Input: part model. Units: mm. Frame: model coordinates. A direction names the side the tool comes from. Coordinates: 2 decimals unless noted, no trailing zeros. Loops run counter-clockwise (first coordinate to the right, second up) from the corner with the lowest first, then second, coordinate; pieces in that order, holes last.
Item 1: Section C-C on z = 1.5. Give the number of separate pieces and of enclosed holes in the cut face, and give its area (3 significant figures).
Item 2: Ray query, line 1 along Z through (x, y) = (10, 0.55) (3 decimals); line 2 along Z through (x, y) = (0, 2.75); line 3 along X through (y, z) = (4.5, 0.75). Return the intervals inside material, ascending.
Item 3: Section D-D on y = 6.5. Return loops of the section in (x, z).
Item 4: Reachability of faces 5 (the flat face through (5, 7, 0)), 6 (the flat face through (0, 5, 2)) from +Z, -Z, +X, -X, +Y, -Y: full face, straight path, thin tool, end or side. Return the list, or none.
Item 5: Pull-direction query (Z, two-part tool) for faces 1 (the flat face through (12.5, 4.54, 1.47)), 2 (the flat face through (5, 3, -5)), 3 (the cylindrical face through (15, 3, 0)), 4 (the flat face through (7.477, 4.535, 1.43)); classes: released by +Z, released by -Z, zero draft, split by the parting line, or undercut.
Item 6: Section A-A on y = 2.25. Return loops of the section in (x, z).
Item 7: Section B-B on x = 9.75. Return loops of the section in (y, z).
Item 8: Contact query for flat-ended pins moving along their axis: P1, Ø1.5, axis at x = 11, y = 4.5, coming from the -Z side; P2, Ø2.5, axis at x = 0, z = 0, coming from the +Y side. Output: stop coordinate, or through.
```python
from build123d import *

# Parameters (mm, degrees)
EXTRUDE_2_DEPTH              = 7
CUT_EXTRUDE_1_DEPTH          = 4
HOLE_WIZARD_M3_1_D           = 3.4
HOLE_WIZARD_M3_1_CSINK_D     = 6.72
HOLE_WIZARD_M3_1_CSINK_ANGLE = 90
HOLE_WIZARD_1_D              = 4.15
HOLE_WIZARD_1_DEPTH          = 10
CUT_EXTRUDE_2_DEPTH          = 5


with BuildPart() as part:
    # 草图1 → 凸台-拉伸2 (new body)
    with BuildSketch(Plane(origin=(0, 0, 0), x_dir=(1, 0, 0), z_dir=(0, 1, 0))):
        with BuildLine():
            Line((0, 5), (10, 5))
            ThreePointArc((10, 5), (15, 0), (10, -5))
            Line((10, -5), (0, -5))
            ThreePointArc((0, -5), (-5, 0), (0, 5))
        make_face()
    extrude(amount=EXTRUDE_2_DEPTH)

    # 草图2 → 切除-拉伸1 (cut)
    with BuildSketch(Plane(origin=(0, 7, 0), x_dir=(1, 0, 0), z_dir=(0, 1, 0))):
        with BuildLine():
            Line((1.5, 2), (-1.5, 2))
            ThreePointArc((-1.5, 2), (-2.5, 0), (-1.5, -2))
            Line((-1.5, -2), (1.5, -2))
            ThreePointArc((1.5, -2), (2.236067977, -1.118033989), (2.5, 0))
            ThreePointArc((2.5, 0), (2.236067977, 1.118033989), (1.5, 2))
        make_face()
    extrude(amount=-CUT_EXTRUDE_1_DEPTH, mode=Mode.SUBTRACT)

    # M3 六角凹锥坑螺钉的锥形沉头孔1 (through all)
    with Locations(Plane(origin=(0, 0, 0), x_dir=(-1, 0, 0), z_dir=(0, -1, 0))):
        with Locations((0, 0)):
            CounterSinkHole(HOLE_WIZARD_M3_1_D / 2, HOLE_WIZARD_M3_1_CSINK_D / 2, counter_sink_angle=HOLE_WIZARD_M3_1_CSINK_ANGLE)

    # 孔1
    with Locations(Plane(origin=(0, 7, 0), x_dir=(1, 0, 0), z_dir=(0, 1, 0))):
        with Locations((10, 0)):
            Hole(HOLE_WIZARD_1_D / 2, depth=HOLE_WIZARD_1_DEPTH)

    # 草图8 → 切除-拉伸2 (cut)
    with BuildSketch(Plane(origin=(0, 7, 0), x_dir=(1, 0, 0), z_dir=(0, 1, 0))):
        Polygon((13.348631561, 0), (11.674315781, 2.9), (8.325684219, 2.9), (6.651368439, 0), (8.325684219, -2.9), (11.674315781, -2.9), align=None)
    extrude(amount=-CUT_EXTRUDE_2_DEPTH, mode=Mode.SUBTRACT)


solid = part.part
```
Results found:
1. separate pieces: 3
1. enclosed holes: 0
1. area: 81.4 mm2
2. line 1: z = -5 to -2.075, 2.075 to 5
2. line 2: z = -5 to -1.7, 1.7 to 5
2. line 3: x = -4.94 to -2.38, 2.38 to 7.08, 12.92 to 14.94
3. outline: (0, -5) - (10, -5) arc R5 ccw to (10, 5) - (0, 5) arc R5 ccw to start; hole (-1.5, -2) - (1.5, -2) arc R2.5 ccw to (1.5, 2) - (-1.5, 2) arc R2.5 ccw to start; hole (6.65, 0) - (8.33, -2.9) - (11.67, -2.9) - (13.35, 0) - (11.67, 2.9) - (8.33, 2.9) - close
4. face 5: +Z, -Z, +X, -X, +Y
4. face 6: +Y
5. face 1: undercut
5. face 2: released by -Z
5. face 3: split by the parting line
5. face 4: undercut
6. outline: (0, -5) - (10, -5) arc R5 ccw to (10, 5) - (0, 5) arc R5 ccw to start; hole circle Ø3.4 at (0, 0); hole (6.65, 0) - (8.33, -2.9) - (11.67, -2.9) - (13.35, 0) - (11.67, 2.9) - (8.33, 2.9) - close
7. outline: (0, -5) - (7, -5) - (7, -2.9) - (2, -2.9) - (2, -2.06) - (0, -2.06) - close; (0, 2.06) - (2, 2.06) - (2, 2.9) - (7, 2.9) - (7, 5) - (0, 5) - close
8. P1: stops at z = -4.99
8. P2: passes through
